The model under review builds one solid part; all positions refer to its coordinate system, in mm. Give positions to 0.01 mm unless a question says otherwise; leave off trailing zeros. Order: outer loops, then holes, each group sorted by start corner. A loop starts at its lowest first (then second) coordinate and runs counter-clockwise, first axis right, second up. Notation, with made-up numbers: (84.5, 7.5) - (93.5, 7.5) arc R6 ccw to (93.5, 11.5) - close; hole circle Ø6 at (5, 70). An arc over 180 degrees is marked (long way). Use CSV: the item, a comma, the result in double quotes. Start each with the question number.
1. Take a section at A-A, the plane y = -89. State the section outline as (x, z) points.
2. Take a section at B-B, the plane x = -25.5. State the section outline as (y, z) points.
3. To check wall thickness, follow line 1 (Y direction, x = 1, z = 55); line 2 (Y direction, x = 48, z = 27). State the ranges of each line that lie inside material, in increasing order. Write a range as [from, to].
4. For pin 1 (4 mm diameter, centred on x = 28.5, z = 11, fed in from -Y); pin 2 (10 mm diameter, centred on x = -6, z = 8.5, fed in from -Y), all flat-tipped, find the tip position at first contact; note any pin that passes through.
```python
from build123d import *

# Parameters (mm, degrees)
F0_W     = 206.4777240157
F0_H     = 137.3893991113
F1_DEPTH = 100.076
F5_DEPTH = 45.8442839212


with BuildPart() as f1:
    # F0 (on Front) → F1 (new body)
    with BuildSketch(Plane.XZ):
        with Locations((-22.1995897591, 1.5661381185)):
            Rectangle(F0_W, F0_H)
    extrude(amount=F1_DEPTH)

    # F4 (on 3pt) → F5 (cut, through all)
    with BuildSketch(Plane(origin=(19.3784317983, -79.9635175807, 29.1231675703), x_dir=(-0.975040899, -0.208619769, 0.0759805056), z_dir=(-0.2220253257, 0.9161693897, -0.3336740987))):
        Polygon((-63.2392349005, 48.8948148407), (-63.2392349005, -97.3229967698), (148.5239067524, 31.7710361682), align=None)
    extrude(amount=-F5_DEPTH, mode=Mode.SUBTRACT)


solid = f1.part
```
Determined:
1,outline,"(-125.44, -67.13) - (81.04, -67.13) - (81.04, -36.72) - (-79.73, 70.26) - (-125.44, 70.26) - close"
2,outline,"(-100.08, -67.13) - (0, -67.13) - (0, 70.26) - (-75.86, 70.26) - (-100.08, 3.76) - close"
3,line 1,"y = [-74.99, 0]"
3,line 2,"y = [-73.8, 0]"
4,pin 1,"stops at y = -85.23"
4,pin 2,"stops at y = -95.81"
